```python
from build123d import *

# Parameters (mm, degrees)
SKETCH_1_W          = 76
SKETCH_1_H          = 60
SKETCH_1_R          = 1.5
EXTRUDE_1_DEPTH     = 2
SKETCH_2_W          = 60
SKETCH_2_H          = 44
EXTRUDE_2_DEPTH     = 5
SKETCH_3_W          = 12
SKETCH_3_H          = 9
SKETCH_3_W_2        = 9
SKETCH_3_H_2        = 12
SKETCH_3_W_3        = 35
SKETCH_3_H_3        = 5
SKETCH_3_W_4        = 5
SKETCH_3_H_4        = 10
EXTRUDE_3_DEPTH     = 9
SKETCH_4_R          = 1.5
CUT_EXTRUDE_1_DEPTH = 26
SKETCH_5_R          = 1.5
CUT_EXTRUDE_2_DEPTH = 26


with BuildPart() as part:
    # 草图1 → 凸台-拉伸1 (new body)
    with BuildSketch(Plane.XY):
        Rectangle(SKETCH_1_W, SKETCH_1_H)
        with Locations((-32.705, 24.765)):
            Circle(SKETCH_1_R, mode=Mode.SUBTRACT)
        with Locations((32.705, 24.765)):
            Circle(SKETCH_1_R, mode=Mode.SUBTRACT)
        with Locations((-32.705, -24.765)):
            Circle(SKETCH_1_R, mode=Mode.SUBTRACT)
        with Locations((32.705, -24.765)):
            Circle(SKETCH_1_R, mode=Mode.SUBTRACT)
    extrude(amount=EXTRUDE_1_DEPTH)

    # 草图2 → 凸台-拉伸2 (add)
    with BuildSketch(Plane.XY.offset(2)):
        Rectangle(SKETCH_2_W, SKETCH_2_H)
    extrude(amount=EXTRUDE_2_DEPTH)

    # 草图3 → 凸台-拉伸3 (add)
    with BuildSketch(Plane(origin=(0, 0, 0), x_dir=(-1, 0, 0), z_dir=(0, 0, -1))):
        with Locations((-34.5, -17.5)):
            Rectangle(SKETCH_3_W, SKETCH_3_H)
        with Locations((-34.5, -1.5)):
            Rectangle(SKETCH_3_W, SKETCH_3_H)
        with Locations((-34.5, 14.5)):
            Rectangle(SKETCH_3_W, SKETCH_3_H)
        with Locations((-21.5, 26.5)):
            Rectangle(SKETCH_3_W_2, SKETCH_3_H_2)
        with Locations((6.5, 26.5)):
            Rectangle(SKETCH_3_W_2, SKETCH_3_H_2)
        with Locations((11.5, -27.5)):
            Rectangle(SKETCH_3_W_3, SKETCH_3_H_3)
        with Locations((35.5, -17.5)):
            Rectangle(SKETCH_3_W_4, SKETCH_3_H_4)
    extrude(amount=EXTRUDE_3_DEPTH)

    # 草图4 → 切除-拉伸1 (cut)
    with BuildSketch(Plane(origin=(40.5, 0, 0), x_dir=(0, 0, -1), z_dir=(1, 0, 0))):
        with Locations((5.5, -17.5)):
            Circle(SKETCH_4_R)
        with Locations((5.5, -1.5)):
            Circle(SKETCH_4_R)
        with Locations((5.5, 14.5)):
            Circle(SKETCH_4_R)
    extrude(amount=-CUT_EXTRUDE_1_DEPTH, mode=Mode.SUBTRACT)

    # 草图5 → 切除-拉伸2 (cut)
    with BuildSketch(Plane(origin=(0, 32.5, 0), x_dir=(1, 0, 0), z_dir=(0, 1, 0))):
        with Locations(Location((21.5, 5.5, 0), (0, 0, 270))):
            Circle(SKETCH_5_R)
        with Locations(Location((-6.5, 5.5, 0), (0, 0, 270))):
            Circle(SKETCH_5_R)
    extrude(amount=-CUT_EXTRUDE_2_DEPTH, mode=Mode.SUBTRACT)


solid = part.part
```
For this review, take the finished solid that the model builds, in its own axes (mm). A direction names the side the tool comes from. Coordinates: 2 decimals unless noted, no trailing zeros. Loops run counter-clockwise (first coordinate to the right, second up) from the corner with the lowest first, then second, coordinate; pieces in that order, holes last.
1. Add section C-C, the plane x = 33. Give the boundary of the cut face in (y, z), then the cut area to 3 significant figures.
2. For line 1 (Y direction, x = 37.25, z = -5.5); line 2 (X direction, y = 26, z = -5.5); line 3 (Y direction, x = -3.5, z = -3.5), list the stretches that pass through material, from the lowest coordinate up.
3. Insertion check: P1, Ø0.8, axis at x = 38.5, y = 16, coming from the +Z side; P2, Ø1.5, axis at x = -15, z = 4, coming from the +Y side; P3, Ø4, axis at x = 4.5, z = 3.5, coming from the -Y side; P4, Ø3.5, axis at x = 32.705, y = -24.765, coming from the -Z side. Each pin has a flat end and moves straight along its axis. Give the tip position at first contact, or say it passes through.
4. Add section D-D, the plane x = 11.5. Give the boundary of the cut face in (y, z).
5. For faces 1 (the flat face through (38, 0, 1)), 2 (the flat face through (6, -28, -4)), 3 (the flat face through (0, 22, 4)), 4 (the flat face through (-33, -18, -4)), 5 (the flat face through (28.5, -2, -3)), list the 3-axis set-ups (+Z, -Z, +X, -X, +Y, -Y) from which the entire face can be reached by the end or side of a thin tool; tool diameter is ignored.
6. Mouldability with a two-part tool opening along Z and no side actions: class faces 6 (the flat face through (35, 15, -9)), 7 (the flat face through (26, 26, -4)), 8 (the cylindrical face through (22.51, 26.58, -6.61)) as +Z half, -Z half, draft (parallel to the pull), parting line (faces both ways), or undercut.
7. Add section A-A, the plane x = -6.5. Give the boundary of the cut face in (y, z).
8. Add section B-B, the plane y = -17.5. Give the boundary of the cut face in (x, z), then the cut area to 3 significant figures.
Result:
1. outline: (-30, 0) - (-26.24, 0) - (-26.24, 2) - (-30, 2) - close; (-23.29, 0) - (-22, 0) - (-22, -9) - (-13, -9) - (-13, 0) - (-6, 0) - (-6, -9) - (3, -9) - (3, 0) - (10, 0) - (10, -9) - (19, -9) - (19, 0) - (23.29, 0) - (23.29, 2) - (-23.29, 2) - close; (26.24, 0) - (30, 0) - (30, 2) - (26.24, 2) - close; hole circle Ø3 at (-17.5, -5.5); hole circle Ø3 at (-1.5, -5.5); hole circle Ø3 at (14.5, -5.5)
1. area: 330 mm2
2. line 1: y = -22 to -19, -16 to -13, -6 to -3, 0 to 3, 10 to 13, 16 to 19
2. line 2: x = -11 to -8, -5 to -2, 17 to 20, 23 to 26
2. line 3: y = -30 to -25, 20.5 to 32.5
3. P1: stops at z = 0
3. P2: stops at y = 22
3. P3: stops at y = -30
3. P4: stops at z = 0
4. outline: (-30, 0) - (30, 0) - (30, 2) - (22, 2) - (22, 7) - (-22, 7) - (-22, 2) - (-30, 2) - close
5. face 1: +Z, +X, +Y, -Y
5. face 2: -Z, +X, +Y, -Y
5. face 3: +Z, +X, -X, +Y
5. face 4: -Z, +Y, -Y
5. face 5: -Z, -X, +Y, -Y
6. face 6: -Z half
6. face 7: draft
6. face 8: undercut
7. outline: (-30, -9) - (-25, -9) - (-25, 0) - (20.5, 0) - (20.5, -4) - (32.5, -4) - (32.5, 0) - (30, 0) - (30, 2) - (22, 2) - (22, 7) - (-22, 7) - (-22, 2) - (-30, 2) - close; (20.5, -9) - (32.5, -9) - (32.5, -7) - (20.5, -7) - close
8. outline: (-38, -9) - (-33, -9) - (-33, 0) - (28.5, 0) - (28.5, -4) - (40.5, -4) - (40.5, 0) - (38, 0) - (38, 2) - (30, 2) - (30, 7) - (-30, 7) - (-30, 2) - (-38, 2) - close; (28.5, -9) - (40.5, -9) - (40.5, -7) - (28.5, -7) - close
8. area: 569 mm2
